Print and shaded views of the part. All mm, measured from the part's lowest x, y and z. Give positions to 0.01 mm unless a question says otherwise; leave off trailing zeros. Loops run counter-clockwise (first coordinate to the right, second up) from the corner with the lowest first, then second, coordinate; pieces in that order, holes last.
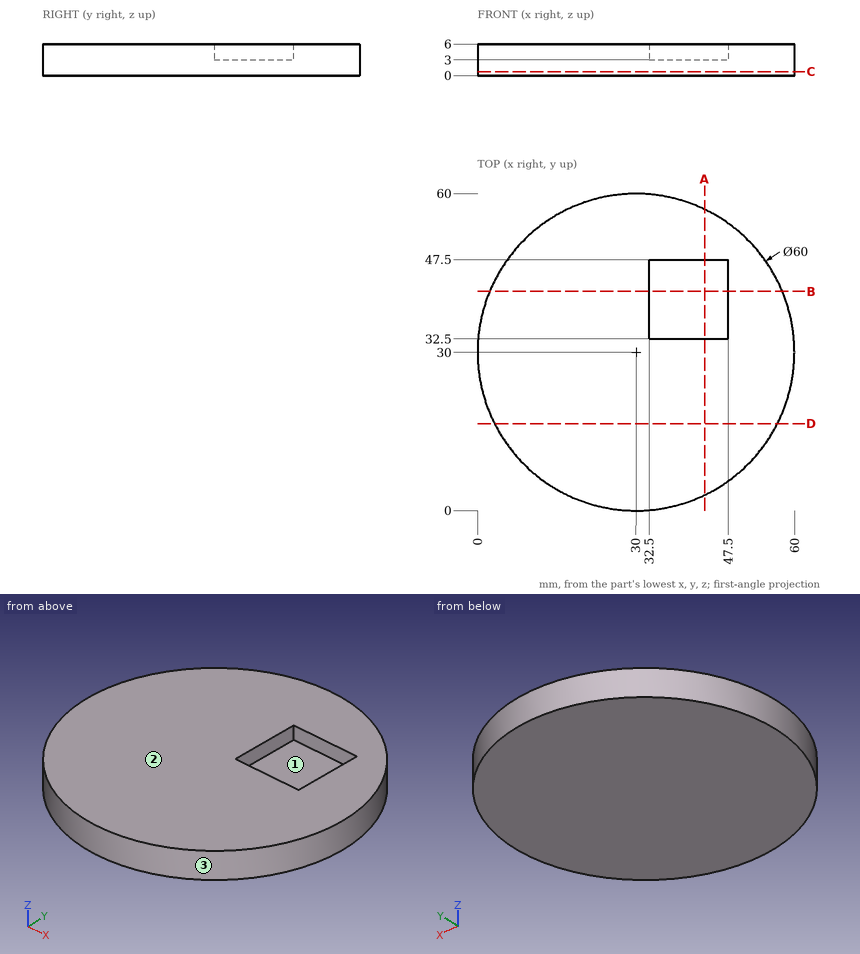
1. Saw through at D-D, the plane y = 16.5. List the corners of the cut face in (x, z), and give its area (3 significant figures).
Responses:
outline: (3.21, 0) - (56.79, 0) - (56.79, 6) - (3.21, 6) - close
area: 321 mm2
2. Probe line 1 along Y through (x, z) = (30, 4.35); line 2 along Y through (x, z) = (40.5, 3.55); line 3 along Z through (x, y) = (38, 35). List the from-to ranges inside material, lowest first.
Responses:
line 1: y = 0 to 60
line 2: y = 1.9 to 32.5, 47.5 to 58.1
line 3: z = 0 to 3
3. Saw through at A-A, the plane x = 43. List the corners of the cut face in (y, z), and give its area (3 significant figures).
Responses:
outline: (2.96, 0) - (57.04, 0) - (57.04, 6) - (47.5, 6) - (47.5, 3) - (32.5, 3) - (32.5, 6) - (2.96, 6) - close
area: 279 mm2
4. Pull direction Y, two halves, no side cores. Call the marked faces 1, 2 and 3: released by +Y, released by -Y, zero draft, split by the parting line, or undercut.
Responses:
face 1: undercut
face 2: zero draft
face 3: split by the parting line
5. Drop flat-ended pins along their axis: pin 1 (1 mm diameter, centred on x = 34.5, z = 1.5, fed in from +Y); pin 2 (2.5 mm diameter, centred on x = 38, z = 5, fed in from -Y); pin 3 (3.5 mm diameter, centred on x = 36.5, z = 4.5, fed in from +Y). Give the stop position or say it passes through.
Responses:
pin 1: stops at y = 59.73
pin 2: stops at y = 0.77
pin 3: stops at y = 59.62
6. Saw through at B-B, the plane y = 41.5. List the corners of the cut face in (x, z).
Responses:
outline: (2.29, 0) - (57.71, 0) - (57.71, 6) - (47.5, 6) - (47.5, 3) - (32.5, 3) - (32.5, 6) - (2.29, 6) - close
7. Saw through at C-C, the plane z = 0.75. List the corners of the cut face in (x, y), and give its area (3 significant figures).
Responses:
outline: circle Ø60 at (30, 30)
area: 2,830 mm2
